Answer from the drawing. Dimensions are ordinates in mm from the lowest x, y and z of the part. A direction names the side the tool comes from. Round coordinates to 2 decimals unless told otherwise and drop trailing zeros. Write each loop counter-clockwise with the first axis right and the second up, starting at its lowest first coordinate (ties: lowest second). Pieces come first, ordered by that corner, then holes.
1. Find section B-B (z = 6.25). Write down the section's boundary in (x, y).
2. Find section A-A (z = 15). Write down the section's boundary in (x, y).
3. A tool of negligible diameter and unlimited length cuts with its end or side. For the marked faces 4 and 5, from which of +Z, -Z, +X, -X, +Y, -Y can it reach the whole face along a straight path? Write none if from no direction.
4. Determine the mould class of the marked faces 1, 2 and 3 for opening direction Y: pulls with the +Y half, pulls with the -Y half, needs draft (parallel to the pull), parting line crosses it, or undercut.
5. Straight lines are drawn through the part: probe 1 along X at (y, z) = (27, 20); probe 2 along Y at (x, z) = (28, 14.7); probe 3 along Y at (x, z) = (28, 21.4). For each, find the intervals that lie inside material, in ascending order.
6. Flat-ended cylindrical pins translate along their axes: pin 1 Ø8 at (x, z) = (32, 3.5) entering from -Y; pin 2 Ø12 at (x, y) = (23, 23.5) entering from -Z; pin 3 Ø19 at (x, y) = (28, 28) entering from -Z. Find the tip coordinate at first contact, or state that the pin passes through.
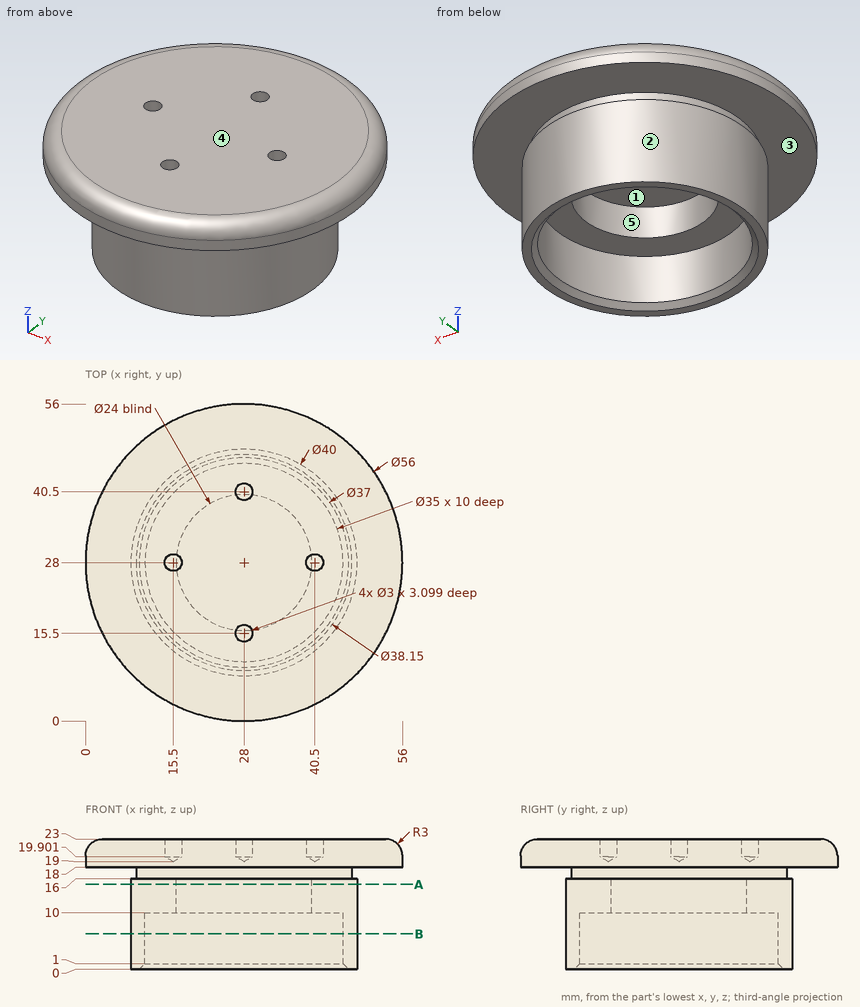
Worked answers:
1. outline: circle Ø40 at (28, 28); hole circle Ø35 at (28, 28)
2. outline: circle Ø40 at (28, 28); hole circle Ø24 at (28, 28)
3. face 4: +Z, +X, -X, +Y, -Y
3. face 5: -Z
4. face 1: undercut
4. face 2: parting line crosses it
4. face 3: needs draft
5. probe 1: x = 0.02 to 14.38, 16.62 to 39.38, 41.62 to 55.98
5. probe 2: y = 8 to 16, 40 to 48
5. probe 3: y = 0.35 to 14, 17 to 39, 42 to 55.65
6. pin 1: stops at y = 8
6. pin 2: stops at z = 10
6. pin 3: stops at z = 16
